For this review, use the dimensioned drawing (mm, ordinates from the lowest corner) and the shaded views. A direction names the side the tool comes from. Coordinates: 2 decimals unless noted, no trailing zeros. Loops run counter-clockwise (first coordinate to the right, second up) from the corner with the lowest first, then second, coordinate; pieces in that order, holes last. Notation, with made-up numbers: (35.5, -15.5) -> (87.5, -15.5) arc R31 cw to (87.5, 14.5) -> close; hole circle Ø6 at (10, 75). An arc over 180 degrees is marked (long way). Answer as a JSON object with one key per item and string values.
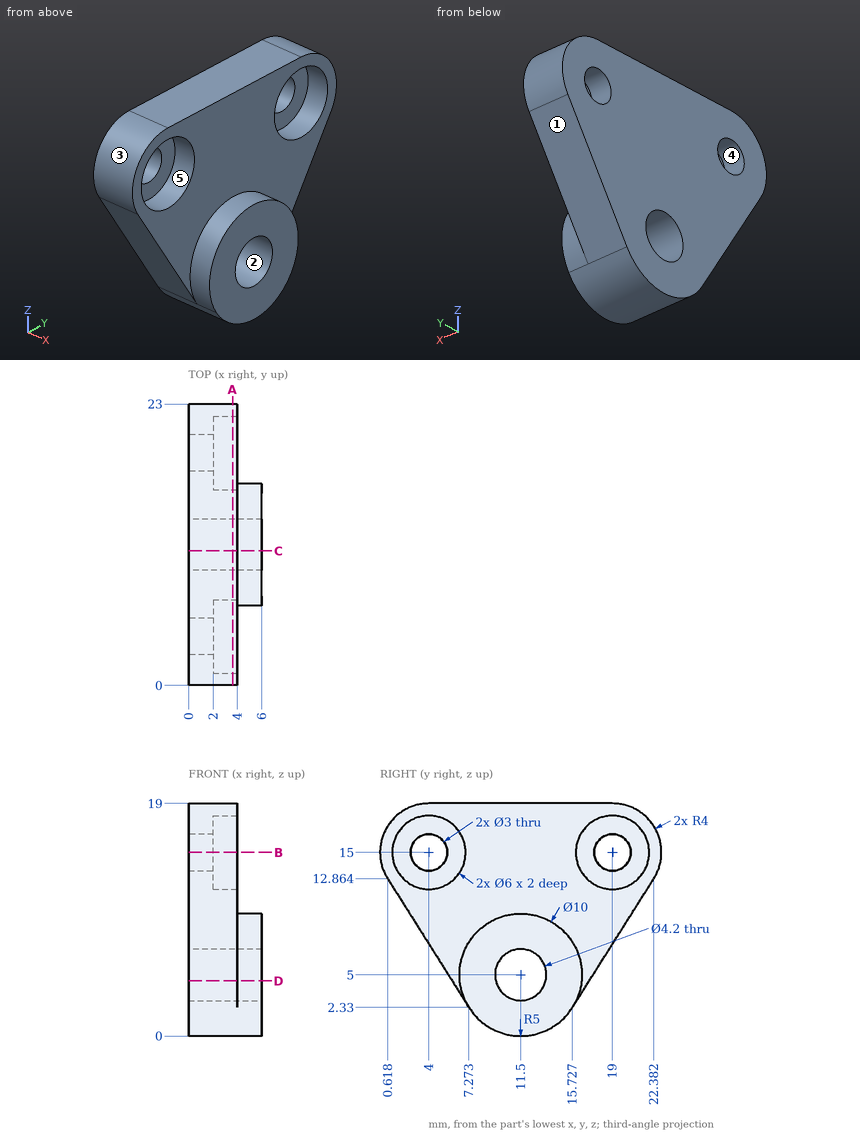
1) The part is to be moulded in two halves that separate along Y. For the marked faces 1, 2 and 3, say which applies: pulls with the +Y half, pulls with the -Y half, needs draft (parallel to the pull), parting line crosses it, or undercut.
Completed:
{"face 1": "pulls with the +Y half", "face 2": "undercut", "face 3": "pulls with the -Y half"}
2) Add section A-A, the plane x = 3.6. Give the boundary of the cut face in (y, z).
Completed:
{"outline": "(0.62, 12.86) -> (7.27, 2.33) arc R5 ccw to (15.73, 2.33) -> (22.38, 12.86) arc R4 ccw to (19, 19) -> (4, 19) arc R4 ccw to start; hole circle Ø6 at (4, 15); hole circle Ø4.2 at (11.5, 5); hole circle Ø6 at (19, 15)"}
3) Wall thickness on probe 1 along Y at (x, z) = (3.3, 15); probe 2 along Y at (x, z) = (1.3, 15); probe 3 along Y at (x, z) = (4.5, 5): over which ranges is each line inside the solid? List them lowest first.
Completed:
{"probe 1": "0 to 1, 7 to 16, 22 to 23", "probe 2": "0 to 2.5, 5.5 to 17.5, 20.5 to 23", "probe 3": "6.5 to 9.4, 13.6 to 16.5"}
4) For the marked faces 4 and 5, list the 3-axis set-ups (+Z, -Z, +X, -X, +Y, -Y) from which the entire face can be reached by the end or side of a thin tool; tool diameter is ignored.
Completed:
{"face 4": "+X, -X", "face 5": "+X"}
5) Add section C-C, the plane y = 11. Give the boundary of the cut face in (x, z) (1 decimal).
Completed:
{"outline": "(0, 0) -> (6, 0) -> (6, 3) -> (0, 3) -> close; (0, 7) -> (6, 7) -> (6, 10) -> (4, 10) -> (4, 19) -> (0, 19) -> close"}
6) Add section B-B, the plane z = 15. Give the boundary of the cut face in (x, y).
Completed:
{"outline": "(0, 0) -> (4, 0) -> (4, 1) -> (2, 1) -> (2, 2.5) -> (0, 2.5) -> close; (0, 5.5) -> (2, 5.5) -> (2, 7) -> (4, 7) -> (4, 16) -> (2, 16) -> (2, 17.5) -> (0, 17.5) -> close; (0, 20.5) -> (2, 20.5) -> (2, 22) -> (4, 22) -> (4, 23) -> (0, 23) -> close"}
7) Add section D-D, the plane z = 4.5. Give the boundary of the cut face in (x, y) (1 decimal).
Completed:
{"outline": "(0, 5.9) -> (4, 5.9) -> (4, 6.5) -> (6, 6.5) -> (6, 9.5) -> (0, 9.5) -> close; (0, 13.5) -> (6, 13.5) -> (6, 16.5) -> (4, 16.5) -> (4, 17.1) -> (0, 17.1) -> close"}
8) Clearance check with flat-ended pins moving along their axes: pin 1 Ø2.5 at (y, z) = (19, 15) entering from -X; pin 2 Ø5 at (y, z) = (20, 16.5) entering from +X; pin 3 Ø1.8 at (y, z) = (5.5, 14) entering from +X. State where each tip first meets the part, or that it passes through.
Completed:
{"pin 1": "through", "pin 2": "x = 4", "pin 3": "x = 2"}
